Input: part model. Units: mm. Frame: model coordinates. A direction names the side the tool comes from. Give positions to 0.01 mm unless a question says otherwise; leave off trailing zeros. Loops run counter-clockwise (first coordinate to the right, second up) from the corner with the lowest first, then second, coordinate; pieces in that order, holes last. Notation, with made-up numbers: M 44.25,41 L 71.25,41 A27 cw 71.25,76 Z; hole C -8,5 d2. An arc over 180 degrees is marked long. One line per item, written item: value. Start each with the question number.
(1) Access query for faces 1 (the flat face through (20.8, 5.802, 2.7)), 2 (the flat face through (0, 17.802, 5)), 3 (the flat face through (-20.8, 5.802, 2.7)). Directions: +Z, -Z, +X, -X, +Y, -Y. A direction counts if a zero-diameter tool reaches every point of the face in a straight line with its end or side. Return the directions, or none.
(2) Section D-D on z = 9.25. Output: boundary loops of the cut face in (x, y).
(3) Pin query (flat end, axial travel): P1, Ø3, axis at y = 13.5, z = 5.5, coming from the -X side; P2, Ø4, axis at x = -19.5, z = 4, coming from the +Y side; P3, Ø5, axis at x = 1.5, z = 7, coming from the -Y side. Return the tip coordinate at first contact, or that it passes through.
(4) Pull-direction query (Z, two-part tool) for faces 4 (the cylindrical face through (7.89, 18.82, 3.99)), 5 (the cylindrical face through (-17.854, 4.816, 4.324)), 6 (the flat face through (2, 18, 10)), 7 (the flat face through (0, 19.802, 5)); classes: released by +Z, released by -Z, zero draft, split by the parting line, or undercut.
(5) Section C-C on z = 5. Output: boundary loops of the cut face in (x, y).
(6) Section B-B on y = 13. Output: boundary loops of the cut face in (x, z).
(7) Section A-A on x = -9. Output: boundary loops of the cut face in (y, z).
(8) Ray query, line 1 along X through (y, z) = (18.5, 5); line 2 along X through (y, z) = (14.25, 8); line 3 along X through (y, z) = (5.1, 5). Return the intervals inside material, ascending. Write a range as from..to.
Autodesk Inventor part; units mm, degrees
ref_plane "YZ Plane" through (0, 0, 0) normal (1, 0, 0) x (0, 1, 0)
ref_plane "XZ Plane" through (0, 0, 0) normal (0, 1, 0) x (-1, 0, 0)
ref_plane "XY Plane" through (0, 0, 0) normal (0, 0, 1) x (1, 0, 0)
sketch "Sketch1" plane through (0, 0, 0) normal (0, 0, 1) x (1, 0, 0)
  line L0 (-16, 19.8024) -> (16, 19.8024)
  line L1 (16, 19.8024) -> (16, 17.8024)
  line L2 (16, 17.8024) -> (-16, 17.8024)
  line L3 (-16, 17.8024) -> (-16, 19.8024)
  line L4 (-16, 17.8024) -> (-14, 17.8024)
  line L5 (-14, 17.8024) -> (-14, 5.8024)
  line L6 (-14, 5.8024) -> (-16, 5.8024)
  line L7 (-16, 5.8024) -> (-16, 17.8024)
  line L8 (16, 17.8024) -> (14, 17.8024)
  line L9 (14, 17.8024) -> (14, 5.8024)
  line L10 (14, 5.8024) -> (16, 5.8024)
  line L11 (16, 5.8024) -> (16, 17.8024)
  line L12 (-14, 5.8024) -> (-24, 5.8024)
  line L13 (-24, 5.8024) -> (-24, 3.8024)
  line L14 (-24, 3.8024) -> (-14, 3.8024)
  line L15 (-14, 3.8024) -> (-14, 5.8024)
  line L16 (14, 5.8024) -> (24, 5.8024)
  line L17 (24, 5.8024) -> (24, 3.8024)
  line L18 (24, 3.8024) -> (14, 3.8024)
  line L19 (14, 3.8024) -> (14, 5.8024)
  point P0 (0, 0)
  point P1 (0, 19.8024)
  dimension "d0" = 32
  dimension "d1" = 2
  dimension "d2" = 2
  dimension "d3" = 12
  dimension "d4" = 2
  dimension "d5" = 12
  dimension "d6" = 10
  dimension "d7" = 2
  dimension "d8" = 10
  dimension "d9" = 2
extrude "Extrusion1" add sketch "Sketch1" along normal blind 10
sketch "Sketch2" plane through (-16, 19.8024, 0) normal (0, 1, 0) x (1, 0, 0)
  line L0 (32, 0) -> (0, 0)
  line L1 (0, 0) -> (0, -10)
  line L2 (32, -10) -> (0, -10)
  line L3 (32, 0) -> (32, -10)
  line L4 (0, 0) -> (0, -10)
  line L5 (32, 0) -> (32, -10)
  circle A0 centre (7, -5) radius 1.5
  circle A1 centre (25, -5) radius 1.5
  line L6 (2, -10) -> (30, -10)
  line L7 (16, -10) -> (16, 0) construction
  dimension "d12" = 3
  dimension "d13" = 3
  dimension "d14" = 9
  dimension "d15" = 9
extrude "Extrusion2" cut sketch "Sketch2" against normal blind 3 contours A0 | A1
sketch "Sketch3" plane through (-24, 5.8024, 0) normal (0, 1, 0) x (1, 0, 0)
  line L0 (8, -10) -> (8, 0)
  line L1 (8, 0) -> (0, 0)
  line L2 (0, 0) -> (0, -10)
  line L3 (8, -10) -> (0, -10)
  circle A0 centre (4, -5) radius 2.25
  point P0 (24, 0)
  dimension "d18" = 4.5
extrude "Extrusion3" cut sketch "Sketch3" against normal blind 3 contours A0
mirror "Mirror1" about plane through (0, 0, 0) normal (1, 0, 0) of "Extrusion3"
sketch "Sketch4" plane through (14, 3.8024, 0) normal (0, -1, 0) x (1, 0, 0)
  circle A0 centre (6, 5) radius 2.25
  line L0 (0, 0) -> (10, 0)
  line L1 (10, 0) -> (10, 10)
  line L2 (0, 10) -> (10, 10)
  line L3 (0, 0) -> (0, 10)
  circle A1 centre (-34, 5) radius 2.25
  line L4 (-38, 0) -> (-28, 0)
  line L5 (-28, 0) -> (-28, 10)
  line L6 (-38, 10) -> (-28, 10)
  line L7 (-38, 0) -> (-38, 10)
  point P0 (-14, 0)
  dimension "d21" = 40
properties part number "EncoderBracket"
Output values:
1. face 1: +Z, -Z, +X, +Y
1. face 2: +Z, -Z, -Y
1. face 3: +Z, -Z, -X, +Y
2. outline: M -24,3.8 L -14,3.8 L -14,17.8 L 14,17.8 L 14,3.8 L 24,3.8 L 24,5.8 L 16,5.8 L 16,19.8 L -16,19.8 L -16,5.8 L -24,5.8 Z
3. P1: stops at x = -16
3. P2: stops at y = 5.8
3. P3: stops at y = 17.8
4. face 4: undercut
4. face 5: undercut
4. face 6: released by +Z
4. face 7: zero draft
5. outline: M -24,3.8 L -22.25,3.8 L -22.25,5.8 L -24,5.8 Z; M -17.75,3.8 L -14,3.8 L -14,17.8 L -10.5,17.8 L -10.5,19.8 L -16,19.8 L -16,5.8 L -17.75,5.8 Z; M -7.5,17.8 L 7.5,17.8 L 7.5,19.8 L -7.5,19.8 Z; M 10.5,17.8 L 14,17.8 L 14,3.8 L 17.75,3.8 L 17.75,5.8 L 16,5.8 L 16,19.8 L 10.5,19.8 Z; M 22.25,3.8 L 24,3.8 L 24,5.8 L 22.25,5.8 Z
6. outline: M -16,0 L -14,0 L -14,10 L -16,10 Z; M 14,0 L 16,0 L 16,10 L 14,10 Z
7. outline: M 17.8,0 L 19.8,0 L 19.8,3.5 L 17.8,3.5 Z; M 17.8,6.5 L 19.8,6.5 L 19.8,10 L 17.8,10 Z
8. line 1: x = -16..-10.5, -7.5..7.5, 10.5..16
8. line 2: x = -16..-14, 14..16
8. line 3: x = -24..-22.25, -17.75..-14, 14..17.75, 22.25..24
